```python
from build123d import *

# Parameters (mm, degrees)
M3_TAPPED_HOLE2_D          = 2.5
M3_TAPPED_HOLE2_DEPTH      = 7.5
M3_TAPPED_HOLE2_TIP        = 0.751075774
SKETCH4_W                  = 6
SKETCH4_H                  = 16
CUT_EXTRUDE1_DEPTH         = 3.5
SKETCH6_W                  = 1.25
SKETCH6_H                  = 16
M3_TAPPED_HOLE1_AT_2_COUNT = 2
M3_TAPPED_HOLE1_AT_2_PITCH = 5
CUT_EXTRUDE2_DEPTH         = 51.815844075
CUT_EXTRUDE2_DEPTH_BACK    = 51.815844075
SKETCH8_R                  = 2.5


with BuildPart() as part:
    # Sketch1 → Revolve1 (revolve)
    with BuildSketch(Plane.XY):
        Polygon((2.5, 30), (2.5, 0), (0, 0), (0, -45.5), (10, -45.5), (10, 26), (16, 26), (16, 30), align=None)
    revolve(axis=Axis((0, -45.5, 0), (0, 1, 0)))

    # M3 Tapped Hole2
    with Locations(Plane(origin=(0, -45.5, 0), x_dir=(-1, 0, 0), z_dir=(0, -1, 0))):
        with Locations((-3.535533906, 3.535533906), (-3.535533906, -3.535533906), (3.535533906, -3.535533906), (3.535533906, 3.535533906)):
            Hole(M3_TAPPED_HOLE2_D / 2, depth=M3_TAPPED_HOLE2_DEPTH)
            with Locations((0, 0, -(M3_TAPPED_HOLE2_DEPTH + M3_TAPPED_HOLE2_TIP / 2))):  # 118° drill point
                Cone(0, M3_TAPPED_HOLE2_D / 2, M3_TAPPED_HOLE2_TIP, mode=Mode.SUBTRACT)

    # Sketch4 → Cut-Extrude1 (cut)
    with BuildSketch(Plane.ZY.offset(10)):
        with Locations((0, 2.5)):
            Rectangle(SKETCH4_W, SKETCH4_H)
        with BuildLine():
            ThreePointArc((-3, 10.5), (0, 13.5), (3, 10.5))
            Line((3, 10.5), (-3, 10.5))
        make_face()
        with BuildLine():
            Line((-3, -5.5), (3, -5.5))
            ThreePointArc((3, -5.5), (0, -8.5), (-3, -5.5))
        make_face()
    extrude(amount=-CUT_EXTRUDE1_DEPTH, mode=Mode.SUBTRACT)

    # Sketch6 → M3 Tapped Hole1 (revolve, cut)
    with BuildSketch(Plane(origin=(0, 21, 0), x_dir=(0, 1, 0), z_dir=(1, 0, 0))):
        with Locations((0.625, 8)):
            Rectangle(SKETCH6_W, SKETCH6_H)
    m3_tapped_hole1 = revolve(axis=Axis((0, 21, -6.35), (0, 0, 1)), mode=Mode.SUBTRACT)

    # M3 Tapped Hole1 at 2: M3 Tapped Hole1 ×2
    with Locations(*[(0, -i * M3_TAPPED_HOLE1_AT_2_PITCH, 0) for i in range(1, M3_TAPPED_HOLE1_AT_2_COUNT)]):
        add(m3_tapped_hole1, mode=Mode.SUBTRACT)

    # Sketch8 → Cut-Extrude2 (cut, two sides: drawn at the far end of the back side and taken through both)
    with BuildSketch(Plane(origin=(0, 0, 0), x_dir=(0, 0, -1), z_dir=(1, 0, 0)).offset(-CUT_EXTRUDE2_DEPTH_BACK)):
        with Locations((0, -20.5)):
            Circle(SKETCH8_R)
    extrude(amount=CUT_EXTRUDE2_DEPTH + CUT_EXTRUDE2_DEPTH_BACK, mode=Mode.SUBTRACT)


solid = part.part
```
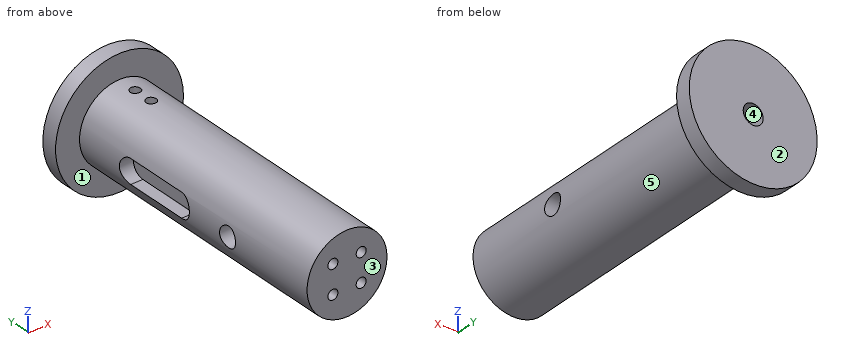
Here's how the part is built. I have some questions about the finished solid (model axes, mm). Face numbers are marked on the shaded views. A direction names the side the tool comes from. Give positions to 0.01 mm unless a question says otherwise; leave off trailing zeros. Write each loop counter-clockwise with the first axis right and the second up, starting at its lowest first coordinate (ties: lowest second). Pieces come first, ordered by that corner, then holes.
(1) Will these pins go through, and if not, where does the flat tip stop? pin 1 (2 mm diameter, centred on y = 8.5, z = -7.5, fed in from -X); pin 2 (1 mm diameter, centred on y = 2, z = 6, fed in from -X); pin 3 (2 mm diameter, centred on y = -18.5, z = -6, fed in from +X); pin 4 (4 mm diameter, centred on y = -20.5, z = 0, fed in from +X).
Output values:
pin 1: stops at x = -7.6
pin 2: stops at x = -8.35
pin 3: stops at x = 8.66
pin 4: passes through
(2) Thinking about a two-plate mould opening in X: for the marked faces 3, 4 and 5, which applies, pulls with the +X half, pulls with the -X half, needs draft (parallel to the pull), parting line crosses it, or undercut?
Output values:
face 3: needs draft
face 4: undercut
face 5: parting line crosses it
(3) Imagine slicing it at A-A, the plane x = 0. Write out the boundary of the cut face in (y, z), and give its area (3 significant figures).
Output values:
outline: (-45.5, -10) - (26, -10) - (26, -16) - (30, -16) - (30, -2.5) - (0, -2.5) - (0, 2.5) - (14.75, 2.5) - (14.75, 10) - (-45.5, 10) - close; (17.25, 2.5) - (19.75, 2.5) - (19.75, 10) - (17.25, 10) - close; (22.25, 2.5) - (30, 2.5) - (30, 16) - (26, 16) - (26, 10) - (22.25, 10) - close; hole circle Ø5 at (-20.5, 0)
area: 1,350 mm2
(4) If I drill on L1, parallel to Y at x = 0, z = 5.25; L2, parallel to X at y = 21, z = 4; L3, parallel to Z at x = -5.25, y = -20.5, over which ranges is the centre line in solid material (lowest first)?
Output values:
L1: y = -45.5 to 14.75, 17.25 to 19.75, 22.25 to 30
L2: x = -9.17 to -1.25, 1.25 to 9.17
L3: z = -8.51 to -2.5, 2.5 to 8.51
(5) On a 3-axis mill with a long thin cutter (end or side, diameter ignored), from which of +Z, -Z, +X, -X, +Y, -Y can I reach the whole of each face in a straight line? I mean the marked faces 1 and 2. Say none if no direction works.
Output values:
face 1: -Y
face 2: +Z, -Z, +X, -X, +Y
(6) Imagine slicing it at C-C, the plane z = 9. Write out the boundary of the cut face in (x, y).
Output values:
outline: (-13.23, 26) - (-4.36, 26) - (-4.36, -45.5) - (4.36, -45.5) - (4.36, 26) - (13.23, 26) - (13.23, 30) - (-13.23, 30) - close; hole circle Ø2.5 at (0, 16); hole circle Ø2.5 at (0, 21)
(7) Imagine slicing it at D-D, the plane y = -21.5. Write out the boundary of the cut face in (x, z), and give its area (3 significant figures).
Output values:
outline: (-9.73, -2.29) arc R10 ccw to (9.73, -2.29) - close; (-9.73, 2.29) - (9.73, 2.29) arc R10 ccw to start
area: 223 mm2
(8) Imagine slicing it at B-B, the plane y = 4.5. Write out the boundary of the cut face in (x, z).
Output values:
outline: (-9.54, -3) arc R10 ccw (long way) to (-9.54, 3) - (-6.5, 3) - (-6.5, -3) - close; hole circle Ø5 at (0, 0)
